Can you work these out from the model? Positions are in its coordinate system, mm. A direction names the side the tool comes from. Give positions to 0.01 mm unless a question says otherwise; leave off trailing zeros. Loops run counter-clockwise (first coordinate to the right, second up) from the corner with the lowest first, then second, coordinate; pieces in that order, holes last. Notation, with made-up numbers: (-13, -35) -> (18, -35) arc R26 cw to (18, -17) -> close; hole circle Ø9 at (-27.75, 75.25). An arc over 180 degrees is marked (long way). One line per question, with ' | ' between items.
from build123d import *

# Parameters (mm, degrees)
F0_R     = 117.5
F1_DEPTH = 220
F1_TAPER = -4
F2_T     = -5
F3_D     = 20
F3_DEPTH = 200
F3_TIP   = 6.0086061903
F5_D     = 150
F5_DEPTH = 125
F5_TIP   = 45.0645464271


with BuildPart() as f1:
    # F0 (on Front) → F1 (new body)
    with BuildSketch(Plane.XZ):
        Circle(F0_R)
    extrude(amount=F1_DEPTH, taper=F1_TAPER)

    # F2
    f2_openings = [f1.faces().sort_by_distance(p)[0] for p in [
        (0, -220, 0),
    ]]
    offset(amount=F2_T, openings=f2_openings, kind=Kind.INTERSECTION)

    # F3
    with Locations(Plane(origin=(0, 0, 0), x_dir=(1, 0, 0), z_dir=(0, 1, 0))):
        with Locations((1.5845698072, 0)):
            Hole(F3_D / 2, depth=F3_DEPTH)
            with Locations((0, 0, -(F3_DEPTH + F3_TIP / 2))):  # 118° drill point
                Cone(0, F3_D / 2, F3_TIP, mode=Mode.SUBTRACT)

    # F5
    with Locations(Plane.XZ.offset(220)):
        with Locations((0, 132.8838986276), (-114.7513767367, -67.0093430165), (114.7513767367, -67.0093430165)):
            Hole(F5_D / 2, depth=F5_DEPTH)
            with Locations((0, 0, -(F5_DEPTH + F5_TIP / 2))):  # 118° drill point
                Cone(0, F5_D / 2, F5_TIP, mode=Mode.SUBTRACT)


solid = f1.part
Q1. If we mould it in two halves opening along Z, with no side actions, what happens to faces 1 (the face through (-111, -220, 67)), 2 (the face through (113.304, -90.116, 35.681)), 3 (the face through (55.67, -156.62, -113.21))? For each: pulls with the +Z half, pulls with the -Z half, needs draft (parallel to the pull), parting line crosses it, or undercut.
Entries:
face 1: needs draft | face 2: undercut | face 3: pulls with the +Z half
Q2. If we section it at C-C (y = -197): Write out the boundary of the cut face in (x, z).
Entries:
outline: (-131.13, 6.18) arc R75 cw to (-126.06, 7.13) arc R126.26 cw to (-69.73, 105.26) arc R75 cw to (-71.46, 110.12) arc R131.28 ccw to start; (-59.06, -117.24) arc R131.28 ccw to (59.06, -117.24) arc R75 cw to (55.74, -113.3) arc R126.26 cw to (-55.74, -113.3) arc R75 cw to start; (69.73, 105.26) arc R126.26 cw to (126.06, 7.13) arc R75 cw to (131.13, 6.18) arc R131.28 ccw to (71.46, 110.12) arc R75 cw to start
Q3. On a 3-axis mill with a long thin cutter (end or side, diameter ignored), from which of +Z, -Z, +X, -X, +Y, -Y can I reach the whole of each face in a straight line? I mean faces 4 (the face through (-125.96, -156.62, 7.15)), 5 (the face through (69.69, -156.63, 105.17)), 6 (the face through (23, -5, 2)), 7 (the face through (-55.553, -156.625, -113.059)). Say none if no direction works.
Entries:
face 4: -Z, -Y | face 5: +Z, -Y | face 6: -Y | face 7: +Z, -X, -Y
Q4. If we section it at B-B (x = 0): Write out the boundary of the cut face in (y, z).
Entries:
outline: (-220, -132.88) -> (0, -117.5) -> (0, -9.87) -> (-5, -9.87) -> (-5, -112.84) -> (-220, -127.87) -> close; (-59.68, 116.66) -> (-5, 112.84) -> (-5, 9.87) -> (0, 9.87) -> (0, 117.5) -> (-56.79, 121.47) -> close
Q5. If I drill on probe 1 along Y at (x, z) = (-95.5, -3.5); probe 2 along X at (y, z) = (-35.5, -56); probe 3 along Z at (x, y) = (-63, -47), over which ranges is the centre line in solid material (lowest first)? Write a range as from..to.
Entries:
probe 1: -5..0 | probe 2: -106.11..-100.41, 100.41..106.11 | probe 3: -103.06..-97.13, 97.13..103.06
Q6. For pin 1 Ø8 at (y, z) = (-76.5, 35.5) entering from -X; pin 2 Ø8 at (x, y) = (-75, -197) entering from -Z; pin 3 Ø12 at (x, z) = (-47, -25.5) entering from -Y; pin 4 Ø12 at (x, z) = (1.58, 0) entering from +Y, each with a flat end and sliding along its axis, tell me the tip position at first contact or that it passes through.
Entries:
pin 1: x = -118.78 | pin 2: z = 98.48 | pin 3: y = -5 | pin 4: through
Q7. If we section it at A-A (y = -136): Write out the boundary of the cut face in (x, z), plus the area to 3 significant figures.
Entries:
outline: (-126.82, 7.01) arc R75 cw to (-121.76, 7.66) arc R122 cw to (-68.02, 101.28) arc R75 cw to (-70.01, 105.97) arc R127.01 ccw to start; (-56.21, -113.89) arc R127.01 ccw to (56.21, -113.89) arc R75 cw to (53.16, -109.81) arc R122 cw to (-53.16, -109.81) arc R75 cw to start; (68.02, 101.28) arc R122 cw to (121.76, 7.66) arc R75 cw to (126.82, 7.01) arc R127.01 ccw to (70.01, 105.97) arc R75 cw to start | area: 1,720 mm²
Q8. If we section it at D-D (y = -40.5): Write out the boundary of the cut face in (x, z), plus the area to 3 significant figures.
Entries:
outline: circle Ø240.66 at (0, 0); hole circle Ø230.64 at (0, 0) | area: 3,710 mm²
